Check sheet for the modelled part. Datum: model origin and axes. Units: mm. Face numbers are marked on the shaded views. A direction names the side the tool comes from. Coordinates: 2 decimals unless noted, no trailing zeros. Loops run counter-clockwise (first coordinate to the right, second up) from the corner with the lowest first, then second, coordinate; pieces in that order, holes last. Notation, with made-up numbers: M -25,10.5 L -3,10.5 A30 ccw -3,42.5 Z; hole C 26.5,-21 d11. An arc over 180 degrees is marked long. Answer in a Markdown table with one row per item. Add a question column.
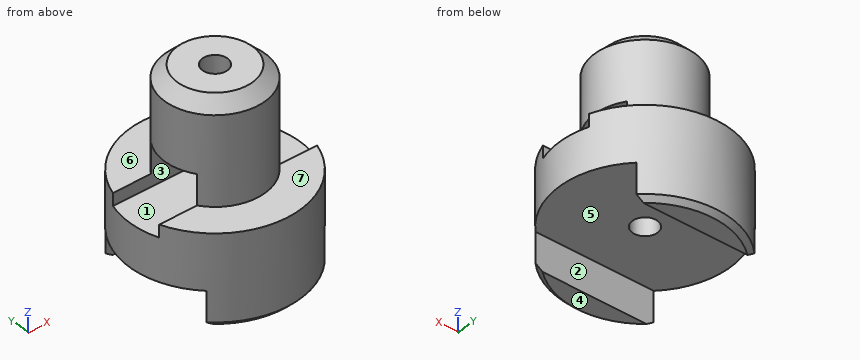
```python
from build123d import *

# Parameters (mm, degrees)
F2_SIZE  = 20
F3_SIZE  = 50
F4_W     = 480
F4_H     = 140
F5_DEPTH = 340
F6_W     = 220
F6_H     = 170
F7_DEPTH = 340
F9_D     = 100


with BuildPart() as f1:
    # F0 (on Front) → F1 (revolve)
    with BuildSketch(Plane.XZ):
        Polygon((0, 0), (0, 760), (-200, 760), (-200, 360), (-340, 360), (-340, 0), align=None)
    revolve(axis=Axis((0, 0, 380), (0, 0, 1)))

    # F2
    f2_edges = [f1.edges().sort_by_distance(p)[0] for p in [
        (340, 0, 0),
    ]]
    chamfer(f2_edges, length=F2_SIZE)

    # F3
    f3_edges = [f1.edges().sort_by_distance(p)[0] for p in [
        (200, 0, 760),
    ]]
    chamfer(f3_edges, length=F3_SIZE)

    # F4 (on Right) → F5 (cut, symmetric)
    with BuildSketch(Plane.YZ):
        with Locations((0, 70)):
            Rectangle(F4_W, F4_H)
    extrude(amount=F5_DEPTH, both=True, mode=Mode.SUBTRACT)

    # F6 (on Right) → F7 (cut, symmetric)
    with BuildSketch(Plane.YZ):
        with Locations((0, 395)):
            Rectangle(F6_W, F6_H)
    extrude(amount=F7_DEPTH, both=True, mode=Mode.SUBTRACT)

    # F9 (through all)
    with Locations(Plane.XY.offset(760)):
        with Locations((0, 0)):
            Hole(F9_D / 2)


solid = f1.part
```
Q1. Cross-section at C-C (z = 194). Record the cut outline in (x, y).
Q2. Go/stop test with flat-tipped pins: pin 1 (10 mm diameter, centred on y = -228.5, z = 175.5, fed in from +X); pin 2 (1.5 mm diameter, centred on x = 91, y = -207, fed in from +Z); pin 3 (3 mm diameter, centred on x = -178, y = 194, fed in from -Z). Record where each tip stops, or that it passes through.
Q3. Cross-section at B-B (x = 0). Record the cut outline in (y, z).
Q4. Access from +Z, -Z, +X, -X, +Y, -Y to the whole of each face (thin tool, end or side, straight path). Record for the marked faces 5, 6 and 7.
Q5. Cross-section at D-D (z = 411). Record the cut outline in (x, y).
Q6. Thickness scan on L1, parallel to Y at x = 0, z = 184; L2, parallel to Z at x = -46, y = 107; L3, parallel to Z at x = 68.5, y = 238.5. Record the ranges inside material, lowest first.
Q7. Cross-section at A-A (y = 0). Record the cut outline in (x, z).
Q8. Mould release check, pull along Z, two halves, no side actions. Record for the marked faces 1, 2, 3 and 4: released by +Z, released by -Z, zero draft, split by the parting line, or undercut.
Answer key:
| question | item | result |
|---|---|---|
| 1 | outline | C 0,0 d680; hole C 0,0 d100 |
| 2 | pin 1 | x = 256.22 |
| 2 | pin 2 | z = 360 |
| 2 | pin 3 | z = 140 |
| 3 | outline | M -340,20 L -320,0 L -240,0 L -240,140 L -50,140 L -50,310 L -110,310 L -110,480 L -50,480 L -50,760 L -150,760 L -200,710 L -200,360 L -340,360 Z; M 50,140 L 240,140 L 240,0 L 320,0 L 340,20 L 340,360 L 200,360 L 200,710 L 150,760 L 50,760 L 50,480 L 110,480 L 110,310 L 50,310 Z |
| 4 | face 5 | -Z, +X, -X |
| 4 | face 6 | +Z, +Y |
| 4 | face 7 | +Z, -Y |
| 5 | outline | M -167.03,-110 A200 ccw 167.03,-110 Z; M -167.03,110 L 167.03,110 A200 ccw Z |
| 6 | L1 | -340 to -50, 50 to 340 |
| 6 | L2 | 140 to 310, 480 to 760 |
| 6 | L3 | 140 to 360 |
| 7 | outline | M -340,140 L -50,140 L -50,310 L -340,310 Z; M -200,480 L -50,480 L -50,760 L -150,760 L -200,710 Z; M 50,140 L 340,140 L 340,310 L 50,310 Z; M 50,480 L 200,480 L 200,710 L 150,760 L 50,760 Z |
| 8 | face 1 | undercut |
| 8 | face 2 | zero draft |
| 8 | face 3 | undercut |
| 8 | face 4 | released by -Z |
